Model file for the job. Use its own axes, mm. A direction names the side the tool comes from. Round coordinates to 2 decimals unless told otherwise and drop trailing zeros. Order: outer loops, then holes, each group sorted by start corner. A loop starts at its lowest first (then second) coordinate and runs counter-clockwise, first axis right, second up. Notation, with made-up numbers: (56.25, 41) - (84.25, 41) arc R24 ccw to (84.25, 68) - close; hole circle Ø1 at (53.25, 18.25). An arc over 180 degrees is marked (long way). Use one line per item in the form item = value.
from build123d import *

# Parameters (mm, degrees)
BLOCK_START            = 303
BLOCK_1_DEPTH          = 240
BLOCK_EDGE_FILLET_1_R  = 6
EXTRUDE_SKETCH_1_W     = 60
EXTRUDE_SKETCH_1_H     = 40
EXTRUDE_1_DEPTH        = 10
EXTRUDE_ROTATE_1_ANGLE = 90


with BuildPart() as part:
    # Block sketch 1 → Block 1 (new body)
    with BuildSketch(Plane.XY.offset(BLOCK_START)):
        with BuildLine():
            Line((684, -115), (831, -115))
            ThreePointArc((831, -115), (840.899494937, -110.899494937), (845, -101))
            Line((845, -101), (845, 101))
            ThreePointArc((845, 101), (840.899494937, 110.899494937), (831, 115))
            Line((831, 115), (684, 115))
            ThreePointArc((684, 115), (674.100505063, 110.899494937), (670, 101))
            Line((670, 101), (670, -101))
            ThreePointArc((670, -101), (674.100505063, -110.899494937), (684, -115))
        make_face()
    extrude(amount=BLOCK_1_DEPTH)

    # Block edge fillet 1
    block_edge_fillet_1_edges = [part.edges().sort_by_distance(p)[0] for p in [
        (845, 0, 303),
        (840.899494937, -110.899494937, 303),
        (757.5, -115, 303),
        (674.100505063, -110.899494937, 303),
        (840.899494937, -110.899494937, 543),
        (845, 0, 543),
        (840.899494937, 110.899494937, 543),
        (757.5, 115, 543),
        (674.100505063, 110.899494937, 543),
        (670, 0, 543),
        (674.100505063, -110.899494937, 543),
        (670, 0, 303),
        (757.5, -115, 543),
        (674.100505063, 110.899494937, 303),
        (757.5, 115, 303),
        (840.899494937, 110.899494937, 303),
    ]]
    fillet(block_edge_fillet_1_edges, radius=BLOCK_EDGE_FILLET_1_R)


with BuildPart() as body_2:
    # Extrude sketch 1 → Extrude 1 (new body)
    with BuildSketch(Plane.XY):
        Rectangle(EXTRUDE_SKETCH_1_W, EXTRUDE_SKETCH_1_H)
    extrude(amount=EXTRUDE_1_DEPTH)


with BuildPart() as body_2_1:
    # Extrude rotate 1: moved
    add(body_2.part.rotate(Axis((0, 0, 0), (0, 1, 0)), EXTRUDE_ROTATE_1_ANGLE))


with BuildPart() as body_2_2:
    # Extrude place 1: moved
    add(body_2_1.part.moved(Location((845, -60, 353))))

    # Combine (weld / assembly of features): union part
    add(part.part)


solid = body_2_2.part
(1) Probe probe 1 along X at (y, z) = (-73.5, 508); probe 2 along Y at (x, z) = (840, 344.5); probe 3 along Y at (x, z) = (836.5, 421). List the from-to ranges inside material, lowest first. Write a range as [from, to].
Report:
probe_1 = [670, 845]
probe_2 = [-111.72, 111.72]
probe_3 = [-113.87, 113.87]
(2) Slice it at B-B on y = 34. Give the cut face in (x, z).
Report:
outline = (670, 309) arc R6 ccw to (676, 303) - (839, 303) arc R6 ccw to (845, 309) - (845, 537) arc R6 ccw to (839, 543) - (676, 543) arc R6 ccw to (670, 537) - close
(3) Slice it at D-D on y = -44. Give the cut face in (x, z), then the cut area to 3 significant figures.
Report:
outline = (670, 309) arc R6 ccw to (676, 303) - (839, 303) arc R6 ccw to (845, 309) - (845, 323) - (855, 323) - (855, 383) - (845, 383) - (845, 537) arc R6 ccw to (839, 543) - (676, 543) arc R6 ccw to (670, 537) - close
area = 42,600 mm2
(4) Slice it at A-A on z = 330. Give the cut face in (x, y).
Report:
outline = (670, -101) arc R14 ccw to (684, -115) - (831, -115) arc R14 ccw to (845, -101) - (845, -80) - (855, -80) - (855, -40) - (845, -40) - (845, 101) arc R14 ccw to (831, 115) - (684, 115) arc R14 ccw to (670, 101) - close
(5) Pin check, flat tips, straight feed: pin 1 (11 mm diameter, centred on x = 852, z = 364, fed in from -Y); pin 2 (1 mm diameter, centred on y = 25, z = 438, fed in from +X); pin 3 (11 mm diameter, centred on x = 848, z = 365.5, fed in from +Y). Stop position of each tip, or through.
Report:
pin_1 = -80
pin_2 = 845
pin_3 = 108.98
(6) Slice it at C-C on z = 478. Give the cut face in (x, y), then the cut area to 3 significant figures.
Report:
outline = (670, -101) arc R14 ccw to (684, -115) - (831, -115) arc R14 ccw to (845, -101) - (845, 101) arc R14 ccw to (831, 115) - (684, 115) arc R14 ccw to (670, 101) - close
area = 40,100 mm2
(7) Tool access for faces 1 (the face through (850, -60, 323)), 2 (the face through (850, -40, 353)), 3 (the face through (759, 115, 421)), 4 (the face through (756, 2, 543)), 5 (the face through (850, -80, 353)): list every direction of +Z, -Z, +X, -X, +Y, -Y with a clear straight run to the whole face (end or side of a thin tool).
Report:
face_1 = -Z, +X, +Y, -Y
face_2 = +Z, -Z, +X, +Y
face_3 = +Z, -Z, +X, -X, +Y
face_4 = +Z, +X, -X, +Y, -Y
face_5 = +Z, -Z, +X, -Y
